Geometry check sheet. Reference: drawing and pictorial views, mm from the part's lowest x, y, z. A direction names the side the tool comes from. Round coordinates to 2 decimals unless told otherwise and drop trailing zeros. Loops run counter-clockwise (first coordinate to the right, second up) from the corner with the lowest first, then second, coordinate; pieces in that order, holes last. Notation, with made-up numbers: (85, -0.75) -> (99, -0.75) arc R24 ccw to (99, 33.25) -> close; hole circle Ø9 at (32.5, 75). An arc over 180 degrees is marked (long way). Use one line per item in the form item = value. Start each with the question number.
(1) Material ranges on probe 1 along Y at (x, z) = (7.5, 9.5); probe 2 along Y at (x, z) = (7.5, 0.1); probe 3 along Y at (x, z) = (7.5, 16.85), recorded low to high. Write a range as [from, to].
(2) Set-up check for the marked faces 3 and 4: record each of +Z, -Z, +X, -X, +Y, -Y from which the full face is reachable in a straight line by a thin tool's end or side.
(3) Draft check along X on the marked faces 1 and 2. Enter one of: released by +X, released by -X, zero draft, split by the parting line, or undercut.
(4) Go/stop test with flat-tipped pins: pin 1 (1 mm diameter, centred on x = 2, y = 10, fed in from +Z); pin 2 (1.5 mm diameter, centred on x = 3, z = 13, fed in from -Y); pin 3 (1 mm diameter, centred on x = 11, z = 7.5, fed in from -Y). Record where each tip stops, or that it passes through.
(5) Sectioned sample at A-A (z = 12). Record the cut outline in (x, y), and give its area (3 significant figures).
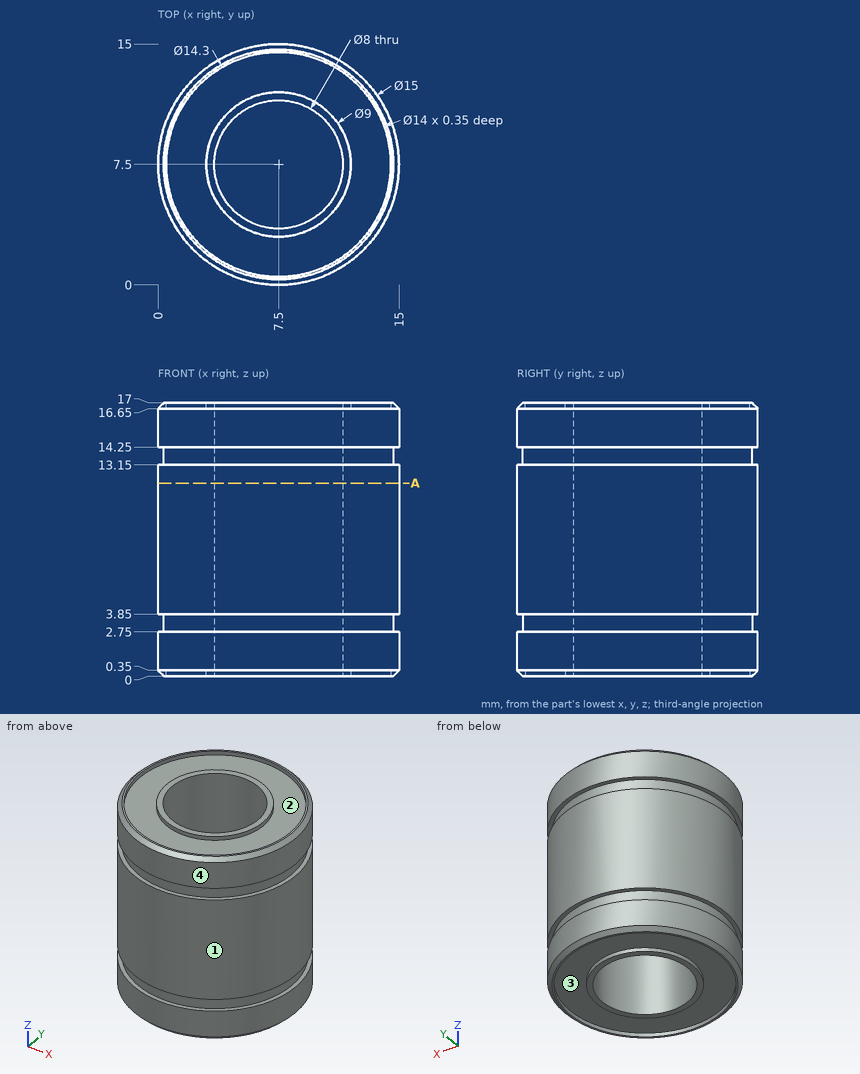
Checks:
q1.probe_1 = [0, 3.5], [11.5, 15]
q1.probe_2 = [0.25, 0.5], [3, 3.5], [11.5, 12], [14.5, 14.75]
q1.probe_3 = [0.2, 0.5], [3, 3.5], [11.5, 12], [14.5, 14.8]
q2.face_3 = -Z
q2.face_4 = +Z, -Z
q3.face_1 = split by the parting line
q3.face_2 = undercut
q4.pin_1 = 16.65
q4.pin_2 = 1
q4.pin_3 = 0.63
q5.outline = circle Ø15 at (7.5, 7.5); hole circle Ø8 at (7.5, 7.5)
q5.area = 126 mm2
